Could you check a few things on this model? Use its own coordinates, in mm. Face numbers are marked on the shaded views. A direction names the side the tool comes from. Round coordinates to 2 decimals unless told otherwise and drop trailing zeros. Loops run counter-clockwise (first coordinate to the right, second up) from the corner with the lowest first, then second, coordinate; pieces in that order, holes last. Notation, with made-up numbers: (51, -27.75) -> (90, -27.75) arc R20 ccw to (90, -4.75) -> close; hole circle Ø7 at (89, 33.25). An arc over 180 degrees is marked (long way). One line per item, written item: value.
```python
from build123d import *

# Parameters (mm, degrees)
F0_W            = 6.35
F0_H            = 22.225
F3_DEPTH        = 6.35
F3_COPIES_COUNT = 8
F4_T1_DEPTH     = 30.2839966419
F4_T3_DEPTH     = 30.283996606
F5_R            = 3.175
F6_DEPTH        = 6.35


# Not quite as in the source:
# - a fillet or chamfer that OpenCascade refuses, or shapes differently, is made with other operations: its cross-section is extruded or revolved along the edge and cut away or added
# - a pattern or mirror of a feature is missing from the dataset's text; its kind, count and spacing are read off the source's solid


with BuildPart() as f1:
    # F0 (on Right) → F1 (revolve)
    with BuildSketch(Plane.YZ):
        with Locations((3.175, 33.3375)):
            Rectangle(F0_W, F0_H)
    revolve(axis=Axis((0, 3.175, 22.225), (0, 1, 0)))

    # F2 (on Front) → F3 (cut)
    with BuildSketch(Plane.XZ):
        with BuildLine():
            Line((-1.59e-08, 38.4876703219), (-1.59e-08, 44.3230155219))
            Line((-1.59e-08, 44.3230155219), (-1.59e-08, 44.457260554))
            Line((-1.59e-08, 44.457260554), (-4.9701853855, 44.457260554))
            Line((-4.9701853855, 44.457260554), (-4.9155350159, 44.3230155219))
            Line((-4.9155350159, 44.3230155219), (-2.8620721488, 39.2788192947))
            ThreePointArc((-2.8620721488, 39.2788192947), (-2.3945935663, 38.7038580036), (-1.6858061527, 38.4876703219))
            Line((-1.6858061527, 38.4876703219), (-1.59e-08, 38.4876703219))
        make_face()
        with BuildLine():
            Line((-1.59e-08, 44.457260554), (-1.59e-08, 44.3230155219))
            Line((-1.59e-08, 44.3230155219), (-1.59e-08, 38.4876703219))
            Line((-1.59e-08, 38.4876703219), (1.6858061209, 38.4876703219))
            ThreePointArc((1.6858061209, 38.4876703219), (2.3945935345, 38.7038580036), (2.8620721171, 39.2788192947))
            Line((2.8620721171, 39.2788192947), (4.9155349841, 44.3230155219))
            Line((4.9155349841, 44.3230155219), (4.9701853538, 44.457260554))
            Line((4.9701853538, 44.457260554), (-1.59e-08, 44.457260554))
        make_face()
    f3 = extrude(amount=-F3_DEPTH, mode=Mode.SUBTRACT)

    # F3_copies: F3 ×8 about axis
    f3_copies_axis = Axis((0, 0, 22.225), (0, 1, 0))
    for i in range(1, F3_COPIES_COUNT):
        add(f3.rotate(f3_copies_axis, i * 360 / F3_COPIES_COUNT), mode=Mode.SUBTRACT)

    # F4: fillet of radius 4.572 on 16 edges, made by hand

    # F4_s2 → F4_t1 (cut)
    with BuildSketch(Plane.XZ.offset(-18.3169983209)):
        with BuildLine():
            ThreePointArc((-3.1489730441, 39.9835724397), (-5.703273274, 42.5117575675), (-9.2958119446, 42.4125829482))
            ThreePointArc((-9.2958119446, 42.4125829482), (-7.0677616426, 43.2962451071), (-4.757507246, 43.934830718))
            Line((-4.757507246, 43.934830718), (-3.1489730441, 39.9835724397))
        make_face()
        with BuildLine():
            ThreePointArc((-10.330546803, 7.4411328104), (-10.3120806372, 3.8472729487), (-7.7016451357, 1.3770915389))
            ThreePointArc((-7.7016451357, 1.3770915389), (-9.901958118, 2.3277175114), (-11.9871028839, 3.5097658457))
            Line((-11.9871028839, 3.5097658457), (-10.330546803, 7.4411328104))
        make_face()
        with BuildLine():
            ThreePointArc((3.1489730441, 4.4664275603), (5.703273274, 1.9382424325), (9.2958119446, 2.0374170518))
            ThreePointArc((9.2958119446, 2.0374170518), (7.0677616426, 1.1537548929), (4.757507246, 0.515169282))
            Line((4.757507246, 0.515169282), (3.1489730441, 4.4664275603))
        make_face()
        with BuildLine():
            ThreePointArc((14.7838671896, 11.894453197), (18.3777270513, 11.9129193628), (20.8479084611, 14.5233548643))
            ThreePointArc((20.8479084611, 14.5233548643), (19.8972824886, 12.323041882), (18.7152341543, 10.2378971161))
            Line((18.7152341543, 10.2378971161), (14.7838671896, 11.894453197))
        make_face()
        with BuildLine():
            ThreePointArc((17.7585724397, 25.3739730441), (20.2867575675, 27.928273274), (20.1875829482, 31.5208119446))
            ThreePointArc((20.1875829482, 31.5208119446), (21.0712451071, 29.2927616426), (21.709830718, 26.982507246))
            Line((21.709830718, 26.982507246), (17.7585724397, 25.3739730441))
        make_face()
        with BuildLine():
            ThreePointArc((10.330546803, 37.0088671896), (10.3120806372, 40.6027270513), (7.7016451357, 43.0729084611))
            ThreePointArc((7.7016451357, 43.0729084611), (9.901958118, 42.1222824886), (11.9871028839, 40.9402341543))
            Line((11.9871028839, 40.9402341543), (10.330546803, 37.0088671896))
        make_face()
        with BuildLine():
            ThreePointArc((-14.7838671896, 32.555546803), (-18.3777270513, 32.5370806372), (-20.8479084611, 29.9266451357))
            ThreePointArc((-20.8479084611, 29.9266451357), (-19.8972824886, 32.126958118), (-18.7152341543, 34.2121028839))
            Line((-18.7152341543, 34.2121028839), (-14.7838671896, 32.555546803))
        make_face()
        with BuildLine():
            ThreePointArc((-17.7585724397, 19.0760269559), (-20.2867575675, 16.521726726), (-20.1875829482, 12.9291880554))
            ThreePointArc((-20.1875829482, 12.9291880554), (-21.0712451071, 15.1572383574), (-21.709830718, 17.467492754))
            Line((-21.709830718, 17.467492754), (-17.7585724397, 19.0760269559))
        make_face()
    extrude(amount=F4_T1_DEPTH, mode=Mode.SUBTRACT)

    # F4_s4 → F4_t3 (cut)
    with BuildSketch(Plane.XZ.offset(-18.316998303)):
        with BuildLine():
            ThreePointArc((9.295811911, 42.4125829637), (5.7032732438, 42.5117575784), (3.1489730174, 39.983572452))
            Line((3.1489730174, 39.983572452), (4.7575072169, 43.9348307244))
            ThreePointArc((4.7575072169, 43.9348307244), (7.0677616109, 43.2962451177), (9.295811911, 42.4125829637))
        make_face()
        with BuildLine():
            ThreePointArc((-9.295811911, 2.0374170363), (-5.7032732438, 1.9382424216), (-3.1489730174, 4.466427548))
            Line((-3.1489730174, 4.466427548), (-4.7575072169, 0.5151692756))
            ThreePointArc((-4.7575072169, 0.5151692756), (-7.0677616109, 1.1537548823), (-9.295811911, 2.0374170363))
        make_face()
        with BuildLine():
            ThreePointArc((7.7016451705, 1.3770915517), (10.3120806663, 3.8472729624), (10.3305468306, 7.4411328206))
            Line((10.3305468306, 7.4411328206), (11.987102909, 3.5097658618))
            ThreePointArc((11.987102909, 3.5097658618), (9.9019581479, 2.3277175263), (7.7016451705, 1.3770915517))
        make_face()
        with BuildLine():
            ThreePointArc((20.1875829637, 12.929188089), (20.2867575784, 16.5217267562), (17.758572452, 19.0760269826))
            Line((17.758572452, 19.0760269826), (21.7098307244, 17.4674927831))
            ThreePointArc((21.7098307244, 17.4674927831), (21.0712451177, 15.1572383891), (20.1875829637, 12.929188089))
        make_face()
        with BuildLine():
            ThreePointArc((20.8479084483, 29.9266451705), (18.3777270376, 32.5370806663), (14.7838671794, 32.5555468306))
            Line((14.7838671794, 32.5555468306), (18.7152341382, 34.212102909))
            ThreePointArc((18.7152341382, 34.212102909), (19.8972824737, 32.1269581479), (20.8479084483, 29.9266451705))
        make_face()
        with BuildLine():
            ThreePointArc((-7.7016451705, 43.0729084483), (-10.3120806663, 40.6027270376), (-10.3305468306, 37.0088671794))
            Line((-10.3305468306, 37.0088671794), (-11.987102909, 40.9402341382))
            ThreePointArc((-11.987102909, 40.9402341382), (-9.9019581479, 42.1222824737), (-7.7016451705, 43.0729084483))
        make_face()
        with BuildLine():
            ThreePointArc((-20.1875829637, 31.520811911), (-20.2867575784, 27.9282732438), (-17.758572452, 25.3739730174))
            Line((-17.758572452, 25.3739730174), (-21.7098307244, 26.9825072169))
            ThreePointArc((-21.7098307244, 26.9825072169), (-21.0712451177, 29.2927616109), (-20.1875829637, 31.520811911))
        make_face()
        with BuildLine():
            ThreePointArc((-20.8479084483, 14.5233548295), (-18.3777270376, 11.9129193337), (-14.7838671794, 11.8944531694))
            Line((-14.7838671794, 11.8944531694), (-18.7152341382, 10.237897091))
            ThreePointArc((-18.7152341382, 10.237897091), (-19.8972824737, 12.3230418521), (-20.8479084483, 14.5233548295))
        make_face()
    extrude(amount=F4_T3_DEPTH, mode=Mode.SUBTRACT)

    # F5 (on Front) → F6 (cut)
    with BuildSketch(Plane.XZ):
        with Locations((0, 22.225)):
            Circle(F5_R)
    extrude(amount=-F6_DEPTH, mode=Mode.SUBTRACT)


solid = f1.part
```
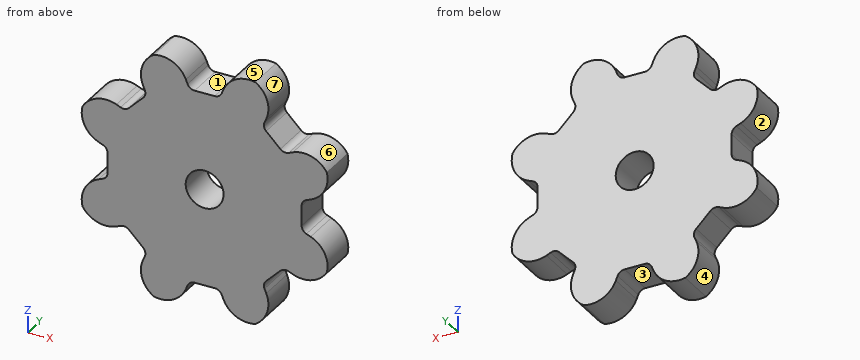
Item 1: I need wall thicknesses on line 1 (Z direction, x = 0, y = 4); line 2 (X direction, y = 5.75, z = 3.5); line 3 (Z direction, x = -2.5, y = 3.75). Which ranges of each line are inside material? Lowest first, please. Write a range as from..to.
Output:
line 1: z = 5.96..19.05, 25.4..38.49
line 2: x = -10.14..-3.69, 3.69..10.14
line 3: z = 5.67..20.27, 24.18..38.78
Item 2: Will these pins go through, and if not, where does the flat tip stop? pin 1 Ø1 at (x, y) = (12.5, 4) entering from -Z; pin 2 Ø2 at (x, y) = (6, 3.5) entering from -Z; pin 3 Ø1.7 at (y, z) = (3, 22) entering from +X; pin 4 Ø4 at (x, z) = (12, 6) entering from -Y.
Output:
pin 1: stops at z = 11.23
pin 2: stops at z = 1.63
pin 3: stops at x = 16.26
pin 4: stops at y = 0
Item 3: If we section it at B-B on z = 18.5: List the corners of the cut face in (x, y) for me.
Output:
outline: (-18.78, 0) -> (18.78, 0) -> (18.78, 6.35) -> (-18.78, 6.35) -> close
Item 4: For the marked faces 1, 2 and 3, which set-ups out of +Z, -Z, +X, -X, +Y, -Y let a thin tool reach every point of the face, with its end or its side?
Output:
face 1: +Z, +Y, -Y
face 2: -X, +Y, -Y
face 3: -Z, +Y, -Y
Item 5: If we section it at A-A on x = 0: List the corners of the cut face in (y, z) for me, plus the area to 3 significant figures.
Output:
outline: (0, 5.96) -> (6.35, 5.96) -> (6.35, 19.05) -> (0, 19.05) -> close; (0, 25.4) -> (6.35, 25.4) -> (6.35, 38.49) -> (0, 38.49) -> close
area: 166 mm²
Item 6: If we section it at C-C on z = 38: List the corners of the cut face in (x, y) for me.
Output:
outline: (-10.62, 0) -> (10.62, 0) -> (10.62, 6.35) -> (-10.62, 6.35) -> close
Item 7: If we mould it in two halves opening along X, with no side actions, what happens to the marked faces 4, 5, 6 and 7? For each: released by +X, released by -X, zero draft, split by the parting line, or undercut.
Output:
face 4: released by -X
face 5: undercut
face 6: undercut
face 7: released by +X
